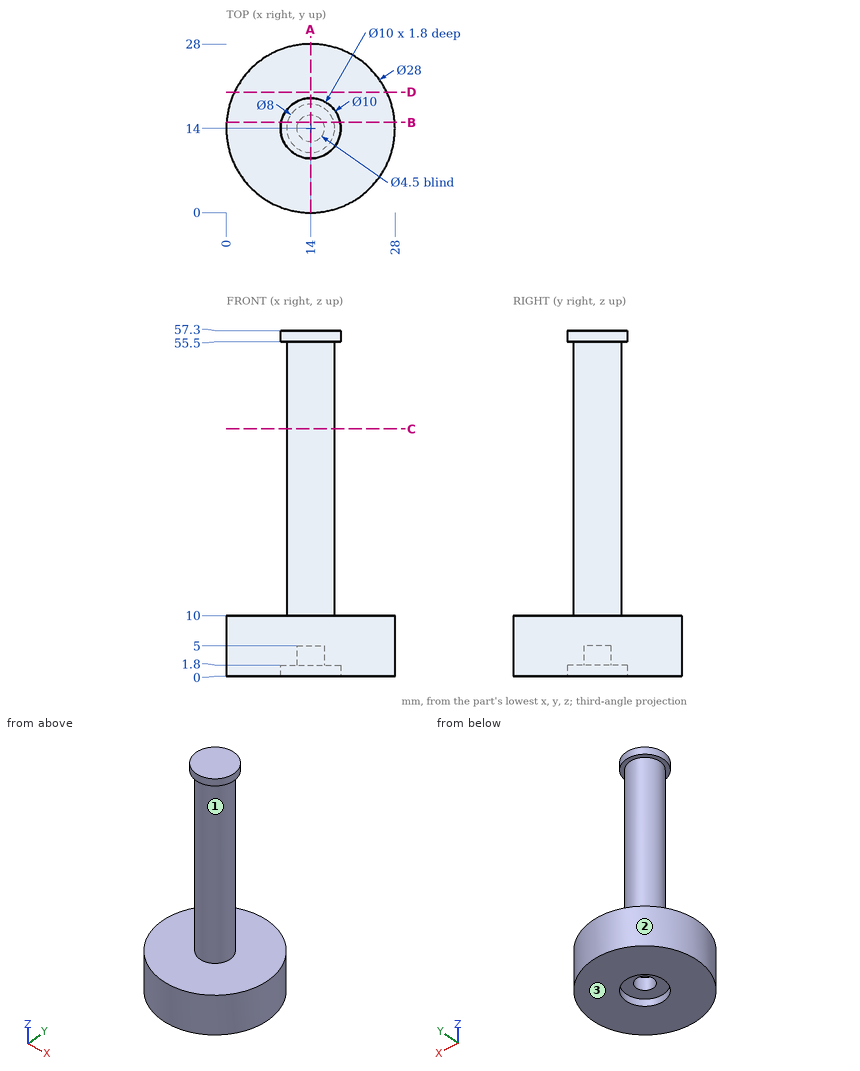
Could you check a few things on this drawing? It's one solid part, dimensions in mm from its lowest x, y, z. Coordinates: 2 decimals unless noted, no trailing zeros. Order: outer loops, then holes, each group sorted by start corner. A loop starts at its lowest first (then second) coordinate and runs counter-clockwise, first axis right, second up. Notation, with made-up numbers: (4.25, -5) - (14.25, -5) arc R18 cw to (14.25, 8) - close; hole circle Ø11 at (-5, 89). An arc over 180 degrees is marked (long way). One line per question, with ' | ' between items.
(1) If I drill on L1, parallel to Y at x = 14, z = 2.55; L2, parallel to Y at x = 14, z = 1.45; L3, parallel to Z at x = 19, y = 24.25, over which ranges is the centre line in solid material (lowest first)?
Report:
L1: y = 0 to 11.75, 16.25 to 28 | L2: y = 0 to 9, 19 to 28 | L3: z = 0 to 10
(2) Suppose I cut it at B-B on y = 15. List the corners of the cut face in (x, z) for me, and give its area (3 significant figures).
Report:
outline: (0.04, 0) - (9.1, 0) - (9.1, 1.8) - (11.98, 1.8) - (11.98, 5) - (16.02, 5) - (16.02, 1.8) - (18.9, 1.8) - (18.9, 0) - (27.96, 0) - (27.96, 10) - (17.87, 10) - (17.87, 55.5) - (18.9, 55.5) - (18.9, 57.3) - (9.1, 57.3) - (9.1, 55.5) - (10.13, 55.5) - (10.13, 10) - (0.04, 10) - close | area: 619 mm2
(3) If we mould it in two halves opening along Z, with no side actions, what happens to the marked faces 1, 2 and 3? For each: pulls with the +Z half, pulls with the -Z half, needs draft (parallel to the pull), parting line crosses it, or undercut.
Report:
face 1: undercut | face 2: needs draft | face 3: pulls with the -Z half
(4) Will these pins go through, and if not, where does the flat tip stop? pin 1 (3 mm diameter, centred on x = 15, y = 15.5, fed in from -Z); pin 2 (5 mm diameter, centred on x = 15, z = 44.5, fed in from -Y); pin 3 (3 mm diameter, centred on x = 10, y = 7.5, fed in from -Z); pin 4 (1.3 mm diameter, centred on x = 13, y = 14.5, fed in from -Z).
Report:
pin 1: stops at z = 1.8 | pin 2: stops at y = 10 | pin 3: stops at z = 0 | pin 4: stops at z = 5
(5) Suppose I cut it at C-C on z = 41. List the corners of the cut face in (x, y) for me, and give its area (3 significant figures).
Report:
outline: circle Ø8 at (14, 14) | area: 50.3 mm2
(6) Suppose I cut it at A-A on x = 14. List the corners of the cut face in (y, z) for me.
Report:
outline: (0, 0) - (9, 0) - (9, 1.8) - (11.75, 1.8) - (11.75, 5) - (16.25, 5) - (16.25, 1.8) - (19, 1.8) - (19, 0) - (28, 0) - (28, 10) - (18, 10) - (18, 55.5) - (19, 55.5) - (19, 57.3) - (9, 57.3) - (9, 55.5) - (10, 55.5) - (10, 10) - (0, 10) - close
(7) Suppose I cut it at D-D on y = 20. List the corners of the cut face in (x, z) for me, and give its area (3 significant figures).
Report:
outline: (1.35, 0) - (26.65, 0) - (26.65, 10) - (1.35, 10) - close | area: 253 mm2
